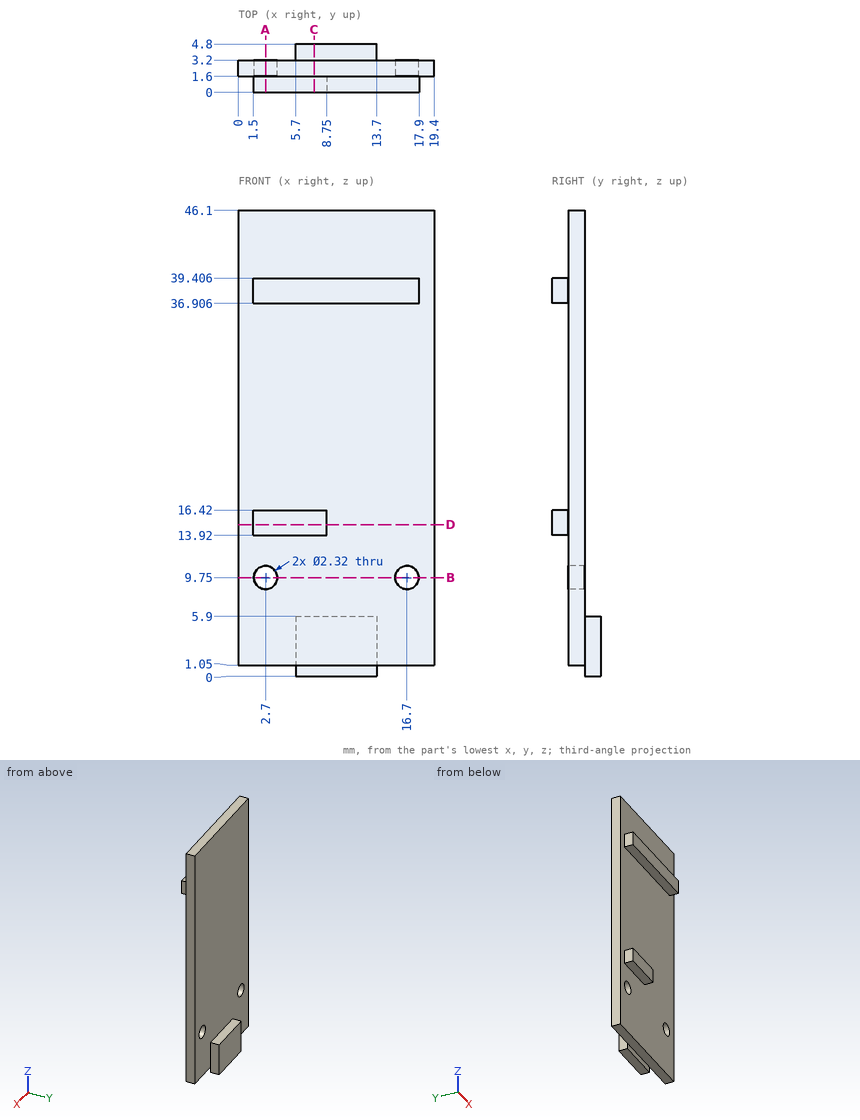
Part print with two shaded views. Sizes in mm from the minimum x, y, z corner. Give positions to 0.01 mm unless a question says otherwise; leave off trailing zeros. Loops run counter-clockwise (first coordinate to the right, second up) from the corner with the lowest first, then second, coordinate; pieces in that order, holes last. Notation, with made-up numbers: (-17.75, 2.5) -> (3.25, 2.5) arc R17 ccw to (3.25, 17.5) -> close; hole circle Ø9 at (-19.5, 8). An arc over 180 degrees is marked (long way). One line per question, with ' | ' between items.
Q1. Drop flat-ended pins along their axis: pin 1 (3.5 mm diameter, centred on x = 2.7, z = 9.75, fed in from +Y); pin 2 (0.8 mm diameter, centred on x = 6, y = 1, fed in from +Z); pin 3 (1.3 mm diameter, centred on x = 10, y = 2, fed in from -Z); pin 4 (1.3 mm diameter, centred on y = 1, z = 37.5, fed in from +X). Give the stop position or say it passes through.
Filled sheet:
pin 1: stops at y = 3.2 | pin 2: stops at z = 39.41 | pin 3: stops at z = 1.05 | pin 4: stops at x = 19.4
Q2. Cut at A-A, the plane x = 2.7. Write the cut outline in (y, z).
Filled sheet:
outline: (0, 13.92) -> (1.6, 13.92) -> (1.6, 10.91) -> (3.2, 10.91) -> (3.2, 46.1) -> (1.6, 46.1) -> (1.6, 39.41) -> (0, 39.41) -> (0, 36.91) -> (1.6, 36.91) -> (1.6, 16.42) -> (0, 16.42) -> close; (1.6, 1.05) -> (3.2, 1.05) -> (3.2, 8.59) -> (1.6, 8.59) -> close
Q3. Cut at D-D, the plane z = 15. Write the cut outline in (x, y).
Filled sheet:
outline: (0, 1.6) -> (1.5, 1.6) -> (1.5, 0) -> (8.75, 0) -> (8.75, 1.6) -> (19.4, 1.6) -> (19.4, 3.2) -> (0, 3.2) -> close
Q4. Cut at B-B, the plane z = 9.75. Write the cut outline in (x, y), plus the area to 3 significant figures.
Filled sheet:
outline: (0, 1.6) -> (1.54, 1.6) -> (1.54, 3.2) -> (0, 3.2) -> close; (3.86, 1.6) -> (15.54, 1.6) -> (15.54, 3.2) -> (3.86, 3.2) -> close; (17.86, 1.6) -> (19.4, 1.6) -> (19.4, 3.2) -> (17.86, 3.2) -> close | area: 23.6 mm²
Q5. Cut at C-C, the plane x = 7.5. Write the cut outline in (y, z).
Filled sheet:
outline: (0, 13.92) -> (1.6, 13.92) -> (1.6, 1.05) -> (3.2, 1.05) -> (3.2, 0) -> (4.8, 0) -> (4.8, 5.9) -> (3.2, 5.9) -> (3.2, 46.1) -> (1.6, 46.1) -> (1.6, 39.41) -> (0, 39.41) -> (0, 36.91) -> (1.6, 36.91) -> (1.6, 16.42) -> (0, 16.42) -> close
Q6. Drill centre lines: line 1 along X through (y, z) = (2.4, 9.75); line 2 along Z through (x, y) = (16.7, 2.7); line 3 along Z through (x, y) = (5.75, 0.2). Where is each one in solid material? Low to high. Write a range as [from, to].
Filled sheet:
line 1: x = [0, 1.54], [3.86, 15.54], [17.86, 19.4] | line 2: z = [1.05, 8.59], [10.91, 46.1] | line 3: z = [13.92, 16.42], [36.91, 39.41]
